Check sheet for the modelled part. Datum: model origin and axes. Units: mm. Round coordinates to 2 decimals unless told otherwise and drop trailing zeros. Write each loop counter-clockwise with the first axis right and the second up, starting at its lowest first coordinate (ties: lowest second). Pieces come first, ordered by that corner, then holes.
Item 1: Cross-section at D-D on z = 10.5. Enter the section's corners in (x, y).
Item 2: Cross-section at A-A on z = 20. Enter the section's corners in (x, y), plus the area to 3 significant figures.
Item 3: Cross-section at B-B on x = -43. Enter the section's corners in (y, z).
Item 4: Cross-section at C-C on y = -59. Enter the section's corners in (x, z), plus the area to 3 significant figures.
Item 5: Material ranges on line 1 (Z direction, x = 47, y = -49); line 2 (Z direction, x = 6.5, y = 46), recorded low to high.
Item 6: Go/stop test with flat-tipped pins: pin 1 Ø10 at (x, y) = (-9.5, -36) entering from +Z; pin 2 Ø1.5 at (x, y) = (3, 25.5) entering from +Z. Record where each tip stops, or that it passes through.
from build123d import *


with BuildPart() as f3:
    # F0 (on Top) → F3 section 0
    with BuildSketch(Plane.XY, mode=Mode.PRIVATE) as f3_s0:
        Polygon((12.097289, 81.748076), (-56.370683, 60.427133), (-82.390381, -6.396673), (-46.368442, -68.403654), (24.56988, -78.901288), (77.006581, -29.984643), (71.455756, 41.51105), align=None)
    loft([Vertex(6.095344, -23.590403, 25.4), f3_s0.sketch])


solid = f3.part
Response values:
1. outline: (-45.81, -13.5) - (-24.68, -49.88) - (16.93, -56.04) - (47.69, -27.34) - (44.44, 14.6) - (9.62, 38.2) - (-30.55, 25.7) - close
2. outline: (-12.72, -19.94) - (-5.06, -33.12) - (10.02, -35.35) - (21.17, -24.95) - (19.99, -9.75) - (7.37, -1.2) - (-7.18, -5.73) - close
2. area: 845 mm2
3. outline: (-68.9, 0) - (64.59, 0) - (42.44, 5.44) - (-14.05, 11.31) - (-65.53, 1.63) - close
4. outline: (-51.83, 0) - (45.9, 0) - (17.92, 9.14) - (-35.36, 5.33) - close
4. area: 557 mm2
5. line 1: z = 0 to 3.14
5. line 2: z = 0 to 8.35
6. pin 1: stops at z = 19.89
6. pin 2: stops at z = 13.31
